The model under review builds one solid part; all positions refer to its coordinate system, in mm. Face numbers are marked on the shaded views. A direction names the side the tool comes from. Round coordinates to 2 decimals unless told otherwise and drop trailing zeros. Write each loop counter-clockwise with the first axis right and the second up, starting at its lowest first coordinate (ties: lowest second). Pieces come first, ordered by that corner, then holes. Notation, with made-up numbers: M -20,51 L -10,51 A29 ccw -10,82 Z; hole C 71.5,78 d2. An arc over 180 degrees is marked long. One line per item, written item: value. Start each with the question number.
1) Take a section at A-A, the plane x = 54. Write out the cut boundary in (y, z), and give its area (3 significant figures).
2) Take a section at C-C, the plane y = -28. Write out the cut boundary in (x, z).
3) Mouldability with a two-part tool opening along Z and no side actions: class the marked faces 3, 4 and 5 as +Z half, -Z half, draft (parallel to the pull), parting line (faces both ways), or undercut.
4) Take a section at D-D, the plane z = 4. Write out the cut boundary in (x, y), and give its area (3 significant figures).
5) Take a section at B-B, the plane z = 0. Write out the cut boundary in (x, y), and give its area (4 significant figures).
6) Tool access review of the marked faces 1 and 2: name each direction out of +Z, -Z, +X, -X, +Y, -Y from which nothing blocks a thin tool from reaching the whole face with its end or side.
7) Wall thickness on probe 1 along Y at (x, z) = (64, -4); probe 2 along Z at (x, y) = (57.5, -4.5); probe 3 along X at (y, z) = (-6.5, 0): over which ranges is each line inside the solid? List them lowest first.
8) For P1, Ø2, axis at x = 22, z = -1.5, coming from the -Y side, flat-tipped, find the tip position at first contact; note if it passes through.
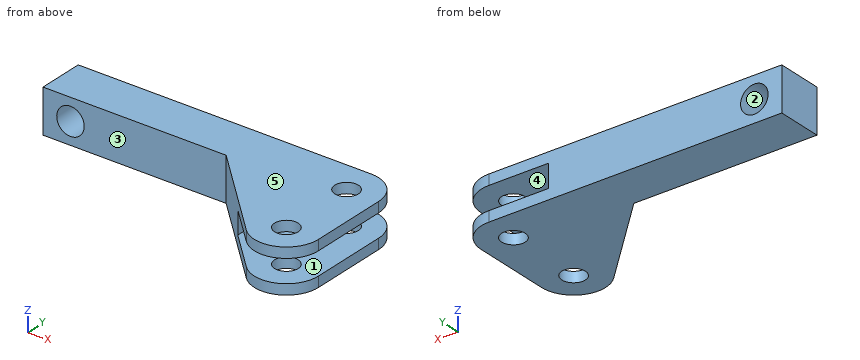
Autodesk Inventor part; units mm, degrees
ref_plane "YZ Plane" through (0, 0, 0) normal (1, 0, 0) x (0, 1, 0)
ref_plane "XZ Plane" through (0, 0, 0) normal (0, 1, 0) x (-1, 0, 0)
ref_plane "XY Plane" through (0, 0, 0) normal (0, 0, 1) x (1, 0, 0)
sketch "Sketch1" plane through (0, 0, 0) normal (0, 0, 1) x (1, 0, 0)
  line L0 (0, 0) -> (64, 0)
  arc A0 (71, -7) -> (64, 0) centre (64, -7) ccw
  line L1 (64, 0) -> (64, -7) construction
  line L2 (71, -7) -> (64, -7) construction
  line L3 (0, 0) -> (0, -10)
  line L4 (0, -10) -> (40, -10)
  line L5 (40, -10) -> (59.0503, -29.0503)
  line L6 (71, -24.1005) -> (71, -7)
  arc A1 (59.0503, -29.0503) -> (71, -24.1005) centre (64, -24.1005) ccw
  line L7 (51, 0) -> (51, -21)
  dimension "d0" = 64
  dimension "d1" = 7
  dimension "d2" = 90
  dimension "d3" = 10
  dimension "d4" = 40
  dimension "d5" = 90
  dimension "d6" = 135
  dimension "d7" = 7
  dimension "d8" = 20
extrude "Extrusion1" add sketch "Sketch1" along normal mid plane 9.525
extrude "Extrusion2" cut sketch "Sketch1" along normal mid plane 5 contours L0 A0 L6 A1 L5 L7
hole "Hole1" at (64, -7, 0) at (64, -24.1005, 0) direction (0, 0, -1) diameter 5.159 end through all both
sketch "Sketch2" plane through (0, 0, -4.7625) normal (0, 1, 0) x (1, 0, 0)
  line L0 (64, -7.2625) -> (51, -7.2625)
  line L1 (51, -7.2625) -> (51, -2.2625)
  line L2 (51, -2.2625) -> (64, -2.2625)
  line L3 (64, -2.2625) -> (64, 0)
  line L4 (0, 0) -> (64, 0)
  line L5 (0, -9.525) -> (0, 0)
  line L6 (64, -9.525) -> (0, -9.525)
  line L7 (64, -9.525) -> (64, -7.2625)
  point P0 (0, -4.7625)
  point P1 (6, -4.7625)
  point P2 (0, -4.7625)
  dimension "d20" = 6
hole "Hole2" at (6, 0, 0) direction (0, -1, 0) diameter 6 end through all
thread "Thread1"
equation "\"d7\" = d1"
properties part number "newfrontpart"
Checked values:
1. outline: M -24,-4.76 L 0,-4.76 L 0,-2.5 L -24,-2.5 Z; M -24,2.5 L 0,2.5 L 0,4.76 L -24,4.76 Z
1. area: 109 mm2
2. outline: M 58,-4.76 L 69.81,-4.76 L 69.81,-2.5 L 58,-2.5 Z; M 58,2.5 L 69.81,2.5 L 69.81,4.76 L 58,4.76 Z
3. face 3: draft
3. face 4: undercut
3. face 5: +Z half
4. outline: M 0,-10 L 40,-10 L 59.05,-29.05 A7 ccw 71,-24.1 L 71,-7 A7 ccw 64,0 L 0,0 Z; hole C 64,-24.1 d5.16; hole C 64,-7 d5.16
4. area: 1,080 mm2
5. outline: M 0,-10 L 3,-10 L 3,0 L 0,0 Z; M 9,-10 L 40,-10 L 51,-21 L 51,0 L 9,0 Z
5. area: 510.5 mm2
6. face 1: +X, +Y, -Y
6. face 2: +Y, -Y
7. probe 1: y = -31.1 to -26.68, -21.52 to -9.58, -4.42 to 0
7. probe 2: z = -4.76 to -2.5, 2.5 to 4.76
7. probe 3: x = 0 to 3, 9 to 51
8. P1: stops at y = -10
